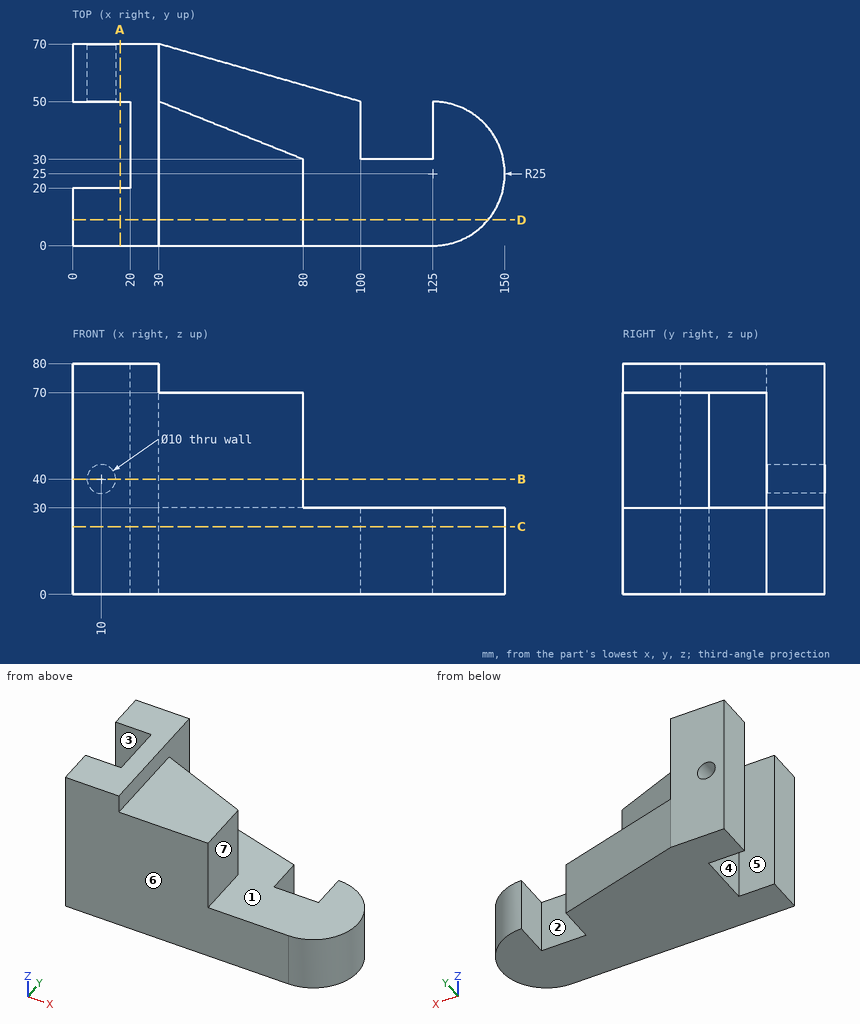
The figure shows three views and two pictorial views of one solid part (mm, origin at its lowest corner). Answer the questions. A direction names the side the tool comes from. Round coordinates to 2 decimals unless told otherwise and drop trailing zeros. Loops run counter-clockwise (first coordinate to the right, second up) from the corner with the lowest first, then second, coordinate; pieces in that order, holes last. Notation, with made-up numbers: M -1.5,51.25 L 57.5,51.25 A23 cw 57.5,74.25 Z; hole C 67,17 d8. An arc over 180 degrees is marked long. Return JSON: item names as keys, results as strings.
Q1. Find the intervals of material crossed by line 1 along Z through (x, y) = (10, 54.25); line 2 along Y through (x, z) = (11.5, 32.5); line 3 along X through (y, z) = (56, 40), in increasing order. Write a range as from..to.
Results list:
{"line 1": "z = 0..35, 45..80", "line 2": "y = 0..20, 50..70", "line 3": "x = 0..5, 15..30"}
Q2. Which of the six approach directions +Z, -Z, +X, -X, +Y, -Y give full straight-line access (tool end or side, diameter ignored) to the marked faces 1, 2 and 3?
Results list:
{"face 1": "+Z, +X, +Y", "face 2": "+Z, -Z, +Y", "face 3": "+Z, -Z, -X"}
Q3. The mould has two halves that part along Y. Classify the marked faces 4, 5, 6 and 7: released by +Y, released by -Y, zero draft, split by the parting line, or undercut.
Results list:
{"face 4": "undercut", "face 5": "undercut", "face 6": "released by -Y", "face 7": "zero draft"}
Q4. Find section B-B, the plane z = 40. Determine the outline of the cut face in (x, y), plus the area to 3 significant figures.
Results list:
{"outline": "M 0,0 L 80,0 L 80,30 L 30,50 L 30,70 L 15,70 L 15,50 L 20,50 L 20,20 L 0,20 Z; M 0,50 L 5,50 L 5,70 L 0,70 Z", "area": "3,300 mm2"}
Q5. Each of these flat-tipped pins is pushed along its axis until it touches: pin 1 Ø12 at (y, z) = (27.5, 39) entering from -X; pin 2 Ø6 at (y, z) = (58, 45.5) entering from -X; pin 3 Ø6 at (y, z) = (45, 10) entering from +X; pin 4 Ø15 at (y, z) = (9, 53) entering from +X. Where does it stop, or does it pass through?
Results list:
{"pin 1": "stops at x = 20", "pin 2": "stops at x = 0", "pin 3": "stops at x = 143.33", "pin 4": "stops at x = 80"}
Q6. Find section C-C, the plane z = 23.5. Determine the outline of the cut face in (x, y), plus the area to 3 significant figures.
Results list:
{"outline": "M 0,0 L 125,0 A25 ccw 125,50 L 125,30 L 100,30 L 100,50 L 30,70 L 0,70 L 0,50 L 20,50 L 20,20 L 0,20 Z", "area": "7,430 mm2"}
Q7. Find section A-A, the plane x = 16.5. Determine the outline of the cut face in (y, z).
Results list:
{"outline": "M 0,0 L 20,0 L 20,80 L 0,80 Z; M 50,0 L 70,0 L 70,80 L 50,80 Z"}
Q8. Find section D-D, the plane y = 9. Determine the outline of the cut face in (x, z).
Results list:
{"outline": "M 0,0 L 144.21,0 L 144.21,30 L 80,30 L 80,70 L 30,70 L 30,80 L 0,80 Z"}
